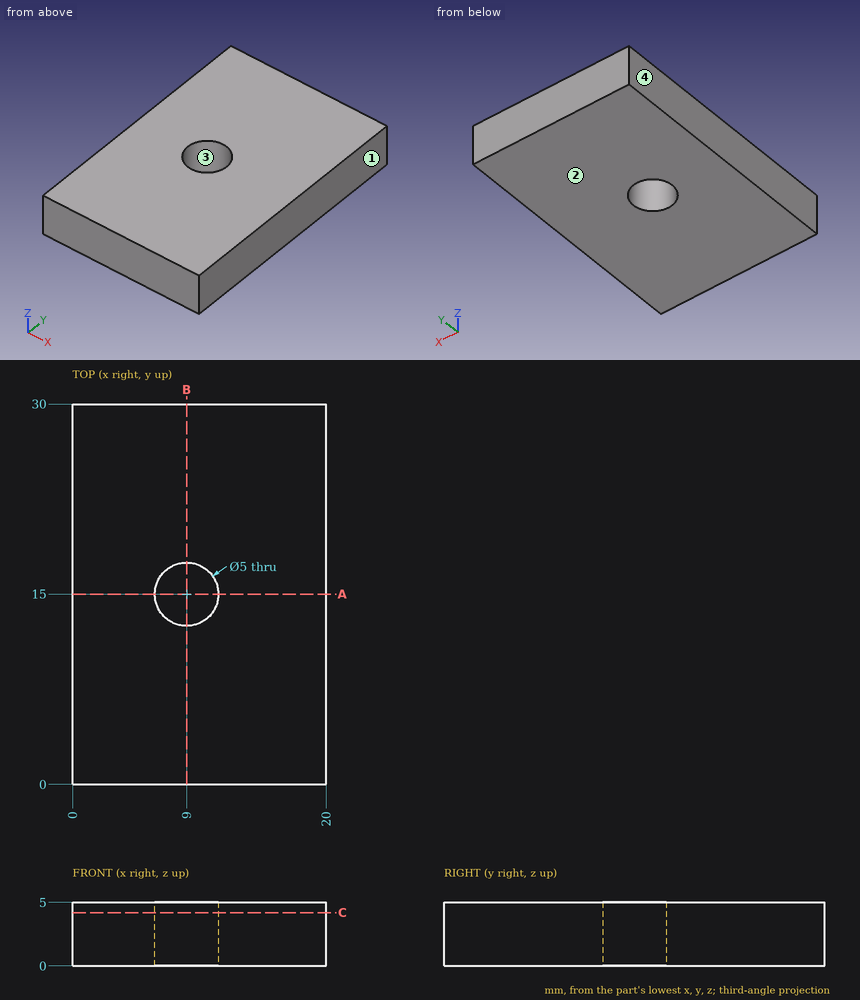
Design review of the part shown in the three views and the two pictorial views. Dimensions are in mm from the part's minimum x, y and z. Coordinates: 2 decimals unless noted, no trailing zeros. Order: outer loops, then holes, each group sorted by start corner. A loop starts at its lowest first (then second) coordinate and runs counter-clockwise, first axis right, second up. Notation, with made-up numbers: (78, 79.25) - (94, 79.25) arc R19 ccw to (94, 93.25) - close; hole circle Ø9 at (65.5, -2). An arc over 180 degrees is marked (long way). One line per question, with ' | ' between items.
Q1. Clearance check with a flat-ended pin moving along its axis: pin 1 Ø6 at (x, y) = (2.5, 16) entering from -Z. State where the tip first meets the part, or that it passes through.
Answer key:
pin 1: stops at z = 0
Q2. Consider section A-A, the plane y = 15. Give the boundary of the cut face in (x, z).
Answer key:
outline: (0, 0) - (6.5, 0) - (6.5, 5) - (0, 5) - close; (11.5, 0) - (20, 0) - (20, 5) - (11.5, 5) - close
Q3. The part is to be moulded in two halves that separate along X. For the marked faces 1, 2, 3 and 4, say which applies: +X half, -X half, draft (parallel to the pull), parting line (faces both ways), or undercut.
Answer key:
face 1: +X half | face 2: draft | face 3: undercut | face 4: -X half
Q4. Consider section B-B, the plane x = 9. Give the boundary of the cut face in (y, z), then the cut area to 3 significant figures.
Answer key:
outline: (0, 0) - (12.5, 0) - (12.5, 5) - (0, 5) - close; (17.5, 0) - (30, 0) - (30, 5) - (17.5, 5) - close | area: 125 mm2
Q5. Consider section C-C, the plane z = 4.2. Give the boundary of the cut face in (x, y), then the cut area to 3 significant figures.
Answer key:
outline: (0, 0) - (20, 0) - (20, 30) - (0, 30) - close; hole circle Ø5 at (9, 15) | area: 580 mm2
Q6. To check wall thickness, follow line 1 along Y through (x, z) = (9, 3.2); line 2 along Y through (x, z) = (11.25, 0.4); line 3 along X through (y, z) = (16, 4.55). State the ranges of each line that lie inside material, in increasing order.
Answer key:
line 1: y = 0 to 12.5, 17.5 to 30 | line 2: y = 0 to 13.91, 16.09 to 30 | line 3: x = 0 to 6.71, 11.29 to 20
